Design review of the part built by this model. Coordinates are the model's own, in mm. A direction names the side the tool comes from. Coordinates: 2 decimals unless noted, no trailing zeros. Loops run counter-clockwise (first coordinate to the right, second up) from the corner with the lowest first, then second, coordinate; pieces in that order, holes last. Notation, with made-up numbers: (33.5, -5.5) - (88.5, -5.5) arc R10 cw to (88.5, 12.5) - close; hole circle Ø10 at (36, 63.25). An arc over 180 degrees is marked (long way). Use one line per item in the form item = value. Start each with the question number.
(1) Clearance check with flat-ended pins moving along their axes: pin 1 Ø2.5 at (x, z) = (19.66, 10.26) entering from +Y; pin 2 Ø0.9 at (x, y) = (27.5, 1) entering from +Z; pin 3 Ø1.5 at (x, y) = (-17.5, 2.5) entering from -Z. State where each tip first meets the part, or that it passes through.
(2) The part is to be moulded in two halves that separate along X. For faces 4 (the face through (15, 1, 20.76)), 5 (the face through (30.576, 1.479, -33.566)), 6 (the face through (-53.33, 1.48, -11.08)), say which applies: pulls with the +X half, pulls with the -X half, needs draft (parallel to the pull), parting line crosses it, or undercut.
(3) Tool access review of faces 1 (the face through (-31.73, 1.48, -16.87)), 2 (the face through (1, 3, -1)), 3 (the face through (-25.33, 1.48, -5.54)): name each direction out of +Z, -Z, +X, -X, +Y, -Y from which nothing blocks a thin tool from reaching the whole face with its end or side.
(4) For L1, parallel to X at y = 1.65, z = -13.5; L2, parallel to X at y = 2.7, z = -10; L3, parallel to Z at x = -51, y = 0.7, list the stretches that pass through material, from the lowest coordinate up.
(5) Add section B-B (z = 18). State the section outline as (x, y) points.
(6) Add section A-A (x = -4). State the section outline as (y, z) points.
```python
from build123d import *

# Parameters (mm, degrees)
EXTRUDE_1_DEPTH     = 3
SKETCH_2_R          = 2
CUT_EXTRUDE_1_DEPTH = 71.204680691


with BuildPart() as part:
    # 草图1 → 凸台-拉伸1 (new body)
    with BuildSketch(Plane(origin=(0, 0, 0), x_dir=(1, 0, 0), z_dir=(0, 1, 0))):
        Polygon((31.465896135, 36.910648046), (32.24235327, 34.012870567), (28.861612878, 33.107003909), (29.896889059, 29.243300604), (30.862814885, 29.502119649), (31.63927202, 26.604342171), (30.673346194, 26.345523125), (32.122732847, 20.936338498), (29.224955368, 20.159881363), (27.775568715, 25.56906599), (26.809642889, 25.310246945), (26.033185754, 28.208024424), (26.99911158, 28.466843469), (25.9638354, 32.330546774), (22.583095008, 31.424680116), (21.806637872, 34.322457595), (-24.55780179, 21.89914343), (-23.781344654, 19.001365951), (-27.162085046, 18.095499294), (-26.126808866, 14.231795988), (-25.16088304, 14.490615033), (-24.384425904, 11.592837555), (-25.350351731, 11.334018509), (-23.900965078, 5.924833882), (-26.798742557, 5.148376747), (-28.248129209, 10.557561374), (-29.214055036, 10.298742329), (-29.990512171, 13.196519808), (-29.024586345, 13.455338853), (-30.059862525, 17.319042158), (-33.440602917, 16.4131755), (-34.217060053, 19.310952979), (-52.569650752, 14.393391122), (-54.11186912, 7.666843213), (-51.214091641, 6.890386078), (-52.119958299, 3.509645686), (-48.140343895, 2.44331122), (-47.88152485, 3.409237046), (-44.983747371, 2.632779911), (-45.242566416, 1.666854085), (-39.833381789, 0.217467432), (-40.609838924, -2.680310047), (-46.019023551, -1.230923394), (-46.277842596, -2.19684922), (-49.175620075, -1.420392085), (-48.91680103, -0.454466259), (-52.780504335, 0.580809922), (-53.686370993, -2.79993047), (-56.584148472, -2.023473335), (-58.137062743, -7.819028293), (-12.738548907, -19.983523413), (-13.515006042, -22.881300891), (-10.617228564, -23.657758027), (-9.840771428, -20.759980548), (40.159228572, -20.759980548), (40.159228572, 39.240019452), align=None)
    extrude(amount=EXTRUDE_1_DEPTH)

    # 草图2 → 切除-拉伸1 (cut, through all)
    with BuildSketch(Plane(origin=(0, 3, 0), x_dir=(1, 0, 0), z_dir=(0, 1, 0))):
        with Locations(Location((19.659228572, -10.259980548, 0), (0, 0, 270))):
            Circle(SKETCH_2_R)
    extrude(amount=-CUT_EXTRUDE_1_DEPTH, mode=Mode.SUBTRACT)


solid = part.part
```
Computed values:
q1.pin_1 = through
q1.pin_2 = 20.76
q1.pin_3 = -23.99
q2.face_4 = needs draft
q2.face_5 = undercut
q2.face_6 = pulls with the -X half
q3.face_1 = -Z, +Y, -Y
q3.face_2 = +Z, -Z, +X, -X, +Y
q3.face_3 = +Y, -Y
q4.L1 = -52.77 to -29.04, -24.9 to 40.16
q4.L2 = -53.58 to -28.1, -24.99 to 40.16
q4.L3 = -14.81 to -3.21, -0.1 to 9.73
q5.outline = (-20.14, 0) - (40.16, 0) - (40.16, 3) - (-20.14, 3) - close
q6.outline = (0, -27.41) - (3, -27.41) - (3, 20.76) - (0, 20.76) - close
